from build123d import *

# Parameters (mm, degrees)
SKETCH1_R           = 2.1
SKETCH1_R_2         = 3.4
BOSS_EXTRUDE1_DEPTH = 255


with BuildPart() as part:
    # Sketch1 → Boss-Extrude1 (new body)
    with BuildSketch(Plane(origin=(0, 0, -1000), x_dir=(-1, 0, 0), z_dir=(0, 0, -1))):
        with BuildLine():
            Line((15, -28), (15, -19.3))
            ThreePointArc((15, -19.3), (14.912132034, -19.087867966), (14.7, -19))
            Line((14.7, -19), (13, -19))
            Line((13, -19), (13, -23.25))
            Line((13, -23.25), (9.6642, -23.25))
            Line((9.6642, -23.25), (6, -19.5858))
            Line((6, -19.5858), (6, -15.519615242))
            Line((6, -15.519615242), (5.7, -15))
            Line((5.7, -15), (6, -14.480384758))
            Line((6, -14.480384758), (6, -10.4142))
            Line((6, -10.4142), (9.6642, -6.75))
            Line((9.6642, -6.75), (13, -6.75))
            Line((13, -6.75), (13, -11))
            Line((13, -11), (14.7, -11))
            ThreePointArc((14.7, -11), (14.912132034, -10.912132034), (15, -10.7))
            Line((15, -10.7), (15, 10.7))
            ThreePointArc((15, 10.7), (14.912132034, 10.912132034), (14.7, 11))
            Line((14.7, 11), (13, 11))
            Line((13, 11), (13, 6.75))
            Line((13, 6.75), (9.6642, 6.75))
            Line((9.6642, 6.75), (6, 10.4142))
            Line((6, 10.4142), (6, 14.480384758))
            Line((6, 14.480384758), (5.7, 15))
            Line((5.7, 15), (6, 15.519615242))
            Line((6, 15.519615242), (6, 19.5858))
            Line((6, 19.5858), (9.6642, 23.25))
            Line((9.6642, 23.25), (13, 23.25))
            Line((13, 23.25), (13, 19))
            Line((13, 19), (14.7, 19))
            ThreePointArc((14.7, 19), (14.912132034, 19.087867966), (15, 19.3))
            Line((15, 19.3), (15, 28))
            ThreePointArc((15, 28), (14.414213562, 29.414213562), (13, 30))
            Line((13, 30), (4.3, 30))
            ThreePointArc((4.3, 30), (4.087867966, 29.912132034), (4, 29.7))
            Line((4, 29.7), (4, 28))
            Line((4, 28), (8.25, 28))
            Line((8.25, 28), (8.25, 24.6642))
            Line((8.25, 24.6642), (4.5858, 21))
            Line((4.5858, 21), (0.519615242, 21))
            Line((0.519615242, 21), (0, 20.7))
            Line((0, 20.7), (-0.519615242, 21))
            Line((-0.519615242, 21), (-4.5858, 21))
            Line((-4.5858, 21), (-8.25, 24.6642))
            Line((-8.25, 24.6642), (-8.25, 28))
            Line((-8.25, 28), (-4, 28))
            Line((-4, 28), (-4, 29.7))
            ThreePointArc((-4, 29.7), (-4.087867966, 29.912132034), (-4.3, 30))
            Line((-4.3, 30), (-13, 30))
            ThreePointArc((-13, 30), (-14.414213562, 29.414213562), (-15, 28))
            Line((-15, 28), (-15, 19.3))
            ThreePointArc((-15, 19.3), (-14.912132034, 19.087867966), (-14.7, 19))
            Line((-14.7, 19), (-13, 19))
            Line((-13, 19), (-13, 23.25))
            Line((-13, 23.25), (-9.6642, 23.25))
            Line((-9.6642, 23.25), (-6, 19.5858))
            Line((-6, 19.5858), (-6, 15.519615242))
            Line((-6, 15.519615242), (-5.7, 15))
            Line((-5.7, 15), (-6, 14.480384758))
            Line((-6, 14.480384758), (-6, 10.4142))
            Line((-6, 10.4142), (-9.6642, 6.75))
            Line((-9.6642, 6.75), (-13, 6.75))
            Line((-13, 6.75), (-13, 11))
            Line((-13, 11), (-14.7, 11))
            ThreePointArc((-14.7, 11), (-14.912132034, 10.912132034), (-15, 10.7))
            Line((-15, 10.7), (-15, -10.7))
            ThreePointArc((-15, -10.7), (-14.912132034, -10.912132034), (-14.7, -11))
            Line((-14.7, -11), (-13, -11))
            Line((-13, -11), (-13, -6.75))
            Line((-13, -6.75), (-9.6642, -6.75))
            Line((-9.6642, -6.75), (-6, -10.4142))
            Line((-6, -10.4142), (-6, -14.480384758))
            Line((-6, -14.480384758), (-5.7, -15))
            Line((-5.7, -15), (-6, -15.519615242))
            Line((-6, -15.519615242), (-6, -19.5858))
            Line((-6, -19.5858), (-9.6642, -23.25))
            Line((-9.6642, -23.25), (-13, -23.25))
            Line((-13, -23.25), (-13, -19))
            Line((-13, -19), (-14.7, -19))
            ThreePointArc((-14.7, -19), (-14.912132034, -19.087867966), (-15, -19.3))
            Line((-15, -19.3), (-15, -28))
            ThreePointArc((-15, -28), (-14.414213562, -29.414213562), (-13, -30))
            Line((-13, -30), (-4.3, -30))
            ThreePointArc((-4.3, -30), (-4.087867966, -29.912132034), (-4, -29.7))
            Line((-4, -29.7), (-4, -28))
            Line((-4, -28), (-8.25, -28))
            Line((-8.25, -28), (-8.25, -24.6642))
            Line((-8.25, -24.6642), (-4.5858, -21))
            Line((-4.5858, -21), (-0.519615242, -21))
            Line((-0.519615242, -21), (0, -20.7))
            Line((0, -20.7), (0.519615242, -21))
            Line((0.519615242, -21), (4.5858, -21))
            Line((4.5858, -21), (8.25, -24.6642))
            Line((8.25, -24.6642), (8.25, -28))
            Line((8.25, -28), (4, -28))
            Line((4, -28), (4, -29.7))
            ThreePointArc((4, -29.7), (4.087867966, -29.912132034), (4.3, -30))
            Line((4.3, -30), (13, -30))
            ThreePointArc((13, -30), (14.414213562, -29.414213562), (15, -28))
        make_face()
        with Locations((11.6, 26.625)):
            Circle(SKETCH1_R, mode=Mode.SUBTRACT)
        with Locations((11.6, -26.625)):
            Circle(SKETCH1_R, mode=Mode.SUBTRACT)
        with Locations((0, -15)):
            Circle(SKETCH1_R_2, mode=Mode.SUBTRACT)
        with Locations((0, 15)):
            Circle(SKETCH1_R_2, mode=Mode.SUBTRACT)
        with Locations((-11.6, 26.625)):
            Circle(SKETCH1_R, mode=Mode.SUBTRACT)
        with Locations((-11.6, -26.625)):
            Circle(SKETCH1_R, mode=Mode.SUBTRACT)
        with BuildLine():
            Line((13, 3.75), (13, -3.75))
            ThreePointArc((13, -3.75), (12.707106781, -4.457106781), (12, -4.75))
            Line((12, -4.75), (8.8358, -4.75))
            Line((8.8358, -4.75), (3.476201279, -10.109598721))
            ThreePointArc((3.476201279, -10.109598721), (0, -9), (-3.476201279, -10.109598721))
            Line((-3.476201279, -10.109598721), (-8.8358, -4.75))
            Line((-8.8358, -4.75), (-12, -4.75))
            ThreePointArc((-12, -4.75), (-12.707106781, -4.457106781), (-13, -3.75))
            Line((-13, -3.75), (-13, 3.75))
            ThreePointArc((-13, 3.75), (-12.707106781, 4.457106781), (-12, 4.75))
            Line((-12, 4.75), (-8.8358, 4.75))
            Line((-8.8358, 4.75), (-3.476201279, 10.109598721))
            ThreePointArc((-3.476201279, 10.109598721), (0, 9), (3.476201279, 10.109598721))
            Line((3.476201279, 10.109598721), (8.8358, 4.75))
            Line((8.8358, 4.75), (12, 4.75))
            ThreePointArc((12, 4.75), (12.707106781, 4.457106781), (13, 3.75))
        make_face(mode=Mode.SUBTRACT)
    extrude(amount=-BOSS_EXTRUDE1_DEPTH)


solid = part.part
Geometry: final body of the model. Coordinates: model frame, mm. A direction names the side the tool comes from. Coordinates: 2 decimals unless noted, no trailing zeros.
1) First-contact query: P1, Ø1.2, axis at y = 13.5, z = -894, coming from the -X side; P2, Ø4.5, axis at y = -17.5, z = -882.5, coming from the +X side; P3, Ø6, axis at x = -0.5, z = -968, coming from the -Y side. Flat tips, straight axial feed; report the tip coordinate or a pass-through.
Result sheet:
P1: stops at x = -6
P2: stops at x = 15
P3: stops at y = -21
2) Set-up query: faces 1 (the flat face through (1, -11, -745)), 2 (the flat face through (-13, 9, -874)). Return all of +Z, -Z, +X, -X, +Y, -Y with unobstructed straight access to the full face (end or side cutting, diameter ignored); none if empty.
Result sheet:
face 1: +Z, +X, -X, +Y, -Y
face 2: +Z, -Z
3) Draft query along X for faces 3 (the flat face through (-15, -24, -874)), 4 (the flat face through (9, 30, -874)), 5 (the flat face through (-6.194, -7.392, -874.285)). Return one class per face: released by +X, released by -X, zero draft, split by the parting line, or undercut.
Result sheet:
face 3: released by -X
face 4: zero draft
face 5: undercut
4) Ray query, probe 1 along Y at (x, z) = (-11.6, -933.5) (3 decimals); probe 2 along X at (y, z) = (19.5, -851.5); probe 3 along X at (y, z) = (20, -977.5). Return the intervals inside material, ascending.
Result sheet:
probe 1: y = -30 to -28.725, -24.525 to -23.25, -6.75 to -4.75, 4.75 to 6.75, 23.25 to 24.525, 28.725 to 30
probe 2: x = -15 to -13, -6 to 6, 13 to 15
probe 3: x = -15 to -13, -6.41 to 6.41, 13 to 15
5) Section A-A (z = -936). Give the number of separate pieces and of enclosed holes in the cut face, then the cut area to 3 significant figures.
Result sheet:
separate pieces: 1
enclosed holes: 7
area: 591 mm2
